Work out the finished part from the listing and answer in its coordinate system (mm). Coordinates: 2 decimals unless noted, no trailing zeros. Answer as a JSON object with one key per item and string values. Group by question number.
Autodesk Inventor part; units mm, degrees
ref_plane "YZ Plane" through (0, 0, 0) normal (1, 0, 0) x (0, 1, 0)
ref_plane "XZ Plane" through (0, 0, 0) normal (0, 1, 0) x (-1, 0, 0)
ref_plane "XY Plane" through (0, 0, 0) normal (0, 0, 1) x (1, 0, 0)
sketch "Sketch1" plane through (0, 0, 0) normal (0, 0, 1) x (1, 0, 0)
  line L0 (-2.55, -10) -> (-2.55, -9.25)
  line L1 (-2.55, -9.25) -> (-2.05, -9.25)
  line L2 (-7.75, -10) -> (-2.55, -10)
  line L3 (-2.05, -9.25) -> (-2.05, -7)
  line L4 (-2.05, -7) -> (-3.05, -7)
  line L5 (-3.05, -9.1) -> (-3.05, -7)
  line L6 (-3.05, -9.1) -> (-5.125, -9.1)
  line L7 (-5.125, -9.1) -> (-5.125, -5.8321)
  line L8 (-8, -9.25) -> (-5.775, -9.25)
  line L9 (-5.775, -9.25) -> (-5.775, -5.775)
  line L10 (-2.2929, -3) -> (2.2929, -3)
  line L11 (3, -2.2929) -> (3, 2.2929)
  line L12 (2.2929, 3) -> (-2.2929, 3)
  line L13 (-3, 2.2929) -> (-3, -2.2929)
  line L14 (-2.2929, -3) -> (-5.125, -5.8321)
  line L15 (-3, -2.2929) -> (-5.8321, -5.125)
  line L16 (-9.1, -5.125) -> (-5.8321, -5.125)
  line L17 (-9.25, -5.775) -> (-5.775, -5.775)
  line L18 (-9.25, -8) -> (-9.25, -5.775)
  line L19 (-10, -7.75) -> (-10, -2.55)
  line L20 (-9.1, -3.05) -> (-9.1, -5.125)
  line L21 (-9.1, -3.05) -> (-7, -3.05)
  line L22 (-9.25, -2.55) -> (-9.25, -2.05)
  line L23 (-9.25, -2.05) -> (-7, -2.05)
  line L24 (-7, -2.05) -> (-7, -3.05)
  line L25 (-10, -2.55) -> (-9.25, -2.55)
  arc A0 (-9.25, -8) -> (-8, -9.25) centre (-8, -8) ccw
  arc A1 (-10, -7.75) -> (-7.75, -10) centre (-7.75, -7.75) ccw
  line L26 (3, -2.2929) -> (5.8321, -5.125)
  line L27 (2.2929, -3) -> (5.125, -5.8321)
  line L28 (5.775, -9.25) -> (5.775, -5.775)
  line L29 (8, -9.25) -> (5.775, -9.25)
  line L30 (7.75, -10) -> (2.55, -10)
  line L31 (3.05, -9.1) -> (5.125, -9.1)
  line L32 (2.55, -10) -> (2.55, -9.25)
  line L33 (3.05, -9.1) -> (3.05, -7)
  line L34 (2.05, -9.25) -> (2.05, -7)
  line L35 (2.55, -9.25) -> (2.05, -9.25)
  line L36 (2.05, -7) -> (3.05, -7)
  line L37 (5.125, -9.1) -> (5.125, -5.8321)
  arc A2 (8, -9.25) -> (9.25, -8) centre (8, -8) ccw
  arc A3 (7.75, -10) -> (10, -7.75) centre (7.75, -7.75) ccw
  line L38 (9.25, -8) -> (9.25, -5.775)
  line L39 (10, -7.75) -> (10, -2.55)
  line L40 (9.25, -5.775) -> (5.775, -5.775)
  line L41 (9.1, -5.125) -> (5.8321, -5.125)
  line L42 (9.1, -3.05) -> (7, -3.05)
  line L43 (7, -2.05) -> (7, -3.05)
  line L44 (9.25, -2.05) -> (7, -2.05)
  line L45 (9.25, -2.55) -> (9.25, -2.05)
  line L46 (10, -2.55) -> (9.25, -2.55)
  line L47 (9.1, -3.05) -> (9.1, -5.125)
  line L48 (2.2929, 3) -> (5.125, 5.8321)
  line L49 (3, 2.2929) -> (5.8321, 5.125)
  line L50 (9.25, 5.775) -> (5.775, 5.775)
  line L51 (9.25, 8) -> (9.25, 5.775)
  line L52 (10, 7.75) -> (10, 2.55)
  line L53 (9.1, 3.05) -> (9.1, 5.125)
  line L54 (10, 2.55) -> (9.25, 2.55)
  line L55 (9.1, 3.05) -> (7, 3.05)
  line L56 (9.25, 2.05) -> (7, 2.05)
  line L57 (9.25, 2.55) -> (9.25, 2.05)
  line L58 (7, 2.05) -> (7, 3.05)
  line L59 (9.1, 5.125) -> (5.8321, 5.125)
  arc A4 (9.25, 8) -> (8, 9.25) centre (8, 8) ccw
  arc A5 (10, 7.75) -> (7.75, 10) centre (7.75, 7.75) ccw
  line L60 (8, 9.25) -> (5.775, 9.25)
  line L61 (7.75, 10) -> (2.55, 10)
  line L62 (5.775, 9.25) -> (5.775, 5.775)
  line L63 (5.125, 9.1) -> (5.125, 5.8321)
  line L64 (3.05, 9.1) -> (3.05, 7)
  line L65 (2.05, 7) -> (3.05, 7)
  line L66 (2.05, 9.25) -> (2.05, 7)
  line L67 (2.55, 9.25) -> (2.05, 9.25)
  line L68 (2.55, 10) -> (2.55, 9.25)
  line L69 (3.05, 9.1) -> (5.125, 9.1)
  line L70 (-3, 2.2929) -> (-5.8321, 5.125)
  line L71 (-2.2929, 3) -> (-5.125, 5.8321)
  line L72 (-5.775, 9.25) -> (-5.775, 5.775)
  line L73 (-8, 9.25) -> (-5.775, 9.25)
  line L74 (-7.75, 10) -> (-2.55, 10)
  line L75 (-3.05, 9.1) -> (-5.125, 9.1)
  line L76 (-2.55, 10) -> (-2.55, 9.25)
  line L77 (-3.05, 9.1) -> (-3.05, 7)
  line L78 (-2.05, 9.25) -> (-2.05, 7)
  line L79 (-2.55, 9.25) -> (-2.05, 9.25)
  line L80 (-2.05, 7) -> (-3.05, 7)
  line L81 (-5.125, 9.1) -> (-5.125, 5.8321)
  arc A6 (-8, 9.25) -> (-9.25, 8) centre (-8, 8) ccw
  arc A7 (-7.75, 10) -> (-10, 7.75) centre (-7.75, 7.75) ccw
  line L82 (-9.25, 8) -> (-9.25, 5.775)
  line L83 (-10, 7.75) -> (-10, 2.55)
  line L84 (-9.25, 5.775) -> (-5.775, 5.775)
  line L85 (-9.1, 5.125) -> (-5.8321, 5.125)
  line L86 (-9.1, 3.05) -> (-7, 3.05)
  line L87 (-7, 2.05) -> (-7, 3.05)
  line L88 (-9.25, 2.05) -> (-7, 2.05)
  line L89 (-9.25, 2.55) -> (-9.25, 2.05)
  line L90 (-10, 2.55) -> (-9.25, 2.55)
  line L91 (-9.1, 3.05) -> (-9.1, 5.125)
  circle A8 centre (0, 0) radius 2
  point P0 (-10, -10)
  point P1 (10, -10)
  point P2 (10, 10)
  point P3 (-10, 10)
  dimension "d2" = 0.75
  dimension "d3" = 7.45
  dimension "d4" = 2.25
  dimension "d5" = 1
  dimension "d6" = 2.1
  dimension "d7" = 0.75
  dimension "d8" = 0.65
  dimension "d9" = 1.25
  dimension "d10" = 2.25
  dimension "d11" = 360
  dimension "d12" = 4
  dimension "d13" = 20
extrude "Extrusion1" add sketch "Sketch1" along normal blind 360
properties part number "2020 dai 360"
Q1. Section A-A on z = 264 is taken. Count the separate pieces of the cut face and the enclosed holes in it, plus the area to 3 significant figures.
Q2. Consider L1, parallel to Y at x = -6.5, z = 59 (3 decimals); L2, parallel to X at y = -7.5, z = 85.5 (3 decimals); L3, parallel to Y at x = 8.25, z = 103 (3 decimals). Determine where each line is inside the solid, lowest interval first. Write a range as from..to.
Q3. Flat-ended cylindrical pins translate along their axes: pin 1 Ø0.8 at (y, z) = (9.5, 213.5) entering from -X; pin 2 Ø1.5 at (x, y) = (-3, -6) entering from -Z; pin 3 Ø1 at (y, z) = (8, 265) entering from -X; pin 4 Ø1 at (x, z) = (-8.5, 124) entering from -Y. Find the tip coordinate at first contact, or state that the pin passes through.
Numbers:
{
 "1": {"separate pieces": "1", "enclosed holes": "5", "area": "117 mm²"},
 "2": {"L1": "y = -10..-9.25, -5.775..-5.125, 5.125..5.775, 9.25..10", "L2": "x = -10..-9.25, -5.775..-5.125, -3.05..-2.05, 2.05..3.05, 5.125..5.775, 9.25..10", "L3": "y = -9.944..-9.225, -5.775..-5.125, -3.05..-2.05, 2.05..3.05, 5.125..5.775, 9.225..9.944"},
 "3": {"pin 1": "stops at x = -9.55", "pin 2": "passes through", "pin 3": "stops at x = -10", "pin 4": "stops at y = -9.99"}
}
